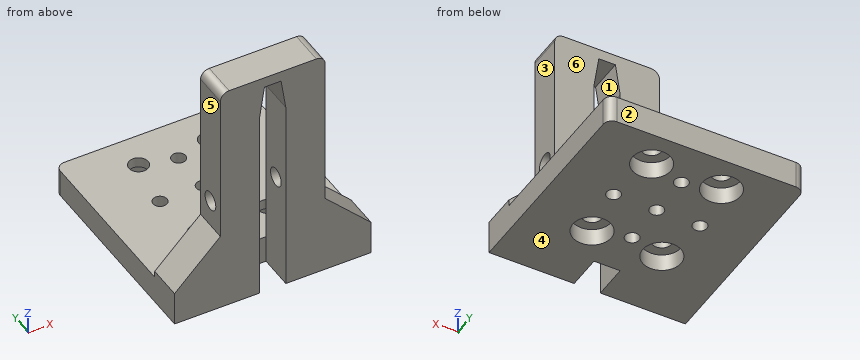
from build123d import *

# Parameters (mm, degrees)
SKETCH1_W                      = 22.5
SKETCH1_H                      = 20
BOSS_EXTRUDE1_DEPTH            = 3.175
TAP_DRILL_FOR_M2X0_4_TAP2_D    = 1.6
BOSS_EXTRUDE2_DEPTH            = 4
CHAMFER1_SIZE                  = 6
M2_CLEARANCE_HOLE1_D           = 2.15
FILLET1_R                      = 1
CBORE_FOR_M2_SHCS1_D           = 2.2
CBORE_FOR_M2_SHCS1_CBORE_D     = 4.4
CBORE_FOR_M2_SHCS1_CBORE_DEPTH = 2


with BuildPart() as part:
    # Sketch1 → Boss-Extrude1 (new body)
    with BuildSketch(Plane.XY):
        Rectangle(SKETCH1_W, SKETCH1_H)
    extrude(amount=BOSS_EXTRUDE1_DEPTH)

    # Tap Drill for M2x0.4 Tap2 (through all)
    with Locations(Plane.XY.offset(3.175)):
        with Locations((0, 0), (-4.949747468, 0), (0, -4.949747468), (4.949747468, 0), (0, 4.949747468)):
            Hole(TAP_DRILL_FOR_M2X0_4_TAP2_D / 2)

    # Sketch10 → Boss-Extrude2 (add)
    with BuildSketch(Plane.XZ.offset(10)):
        Polygon((6, 27.65), (-6, 27.65), (-6, 3.175), (-11.25, 3.175), (-11.25, 0), (-1.5, 0), (-1.5, 22.8), (-0.95, 26.45), (0.95, 26.45), (1.5, 22.8), (1.5, 0), (11.25, 0), (11.25, 3.175), (6, 3.175), align=None)
    extrude(amount=BOSS_EXTRUDE2_DEPTH)

    # Chamfer1
    # the kernel refuses this chamfer: 6 mm, written as the material it adds along each edge
    with BuildSketch(Plane(origin=(-6, -10, 3.175), x_dir=(-0.9996219169112969, 0, -0.02749587661058649), z_dir=(0, -1, 0))) as chamfer1_piece_1_section:
        Polygon((CHAMFER1_SIZE * 0.999621916911, -CHAMFER1_SIZE * 0.0274958766106), (-CHAMFER1_SIZE * 0.0274958766106, -CHAMFER1_SIZE * 0.999621916911), (0, 0), align=None)
    chamfer1_piece_1 = extrude(amount=4, mode=Mode.PRIVATE)
    chamfer1_piece_1 = split(chamfer1_piece_1, bisect_by=Plane(origin=(-11.25, -12, 5.202939), z_dir=(1, 0, 0)), keep=Keep.TOP, mode=Mode.PRIVATE)
    add(chamfer1_piece_1)
    with BuildSketch(Plane(origin=(6, -10, 3.175), x_dir=(0.9996219169112969, 0, -0.02749587661058649), z_dir=(0, -1, 0))) as chamfer1_piece_2_section:
        Polygon((CHAMFER1_SIZE * 0.999621916911, CHAMFER1_SIZE * 0.0274958766106), (-CHAMFER1_SIZE * 0.0274958766106, CHAMFER1_SIZE * 0.999621916911), (0, 0), align=None)
    chamfer1_piece_2 = extrude(amount=4, mode=Mode.PRIVATE)
    chamfer1_piece_2 = split(chamfer1_piece_2, bisect_by=Plane(origin=(11.25, -12, 5.202939), z_dir=(-1, 0, 0)), keep=Keep.TOP, mode=Mode.PRIVATE)
    add(chamfer1_piece_2)

    # M2 Clearance Hole1 (through all)
    with Locations(Plane.ZY.offset(11.25)):
        with Locations((12.35, -12)):
            Hole(M2_CLEARANCE_HOLE1_D / 2)

    # Fillet1
    fillet1_edges = [part.edges().sort_by_distance(p)[0] for p in [
        (6, -12, 27.65),
        (-6, -12, 27.65),
        (-11.25, 10, 1.5875),
        (11.25, 10, 1.5875),
    ]]
    fillet(fillet1_edges, radius=FILLET1_R)

    # CBORE for M2 SHCS1 (through all)
    with Locations(Plane(origin=(0, 0, 0), x_dir=(-1, 0, 0), z_dir=(0, 0, -1))):
        with Locations((4, -6), (-4, 6), (-4, -6), (4, 6)):
            CounterBoreHole(CBORE_FOR_M2_SHCS1_D / 2, CBORE_FOR_M2_SHCS1_CBORE_D / 2, CBORE_FOR_M2_SHCS1_CBORE_DEPTH)


solid = part.part
For this review, take the finished solid that the model builds, in its own axes (mm). Face numbers are marked on the shaded views. A direction names the side the tool comes from. Round coordinates to 2 decimals unless told otherwise and drop trailing zeros. Loops run counter-clockwise (first coordinate to the right, second up) from the corner with the lowest first, then second, coordinate; pieces in that order, holes last. Notation, with made-up numbers: (3.25, -4) - (23.25, -4) arc R11 cw to (23.25, 9) - close; hole circle Ø1 at (55.25, -16.75). An arc over 180 degrees is marked (long way). One line per question, with ' | ' between items.
Q1. The part is to be moulded in two halves that separate along X. For the marked faces 1, 2 and 3, say which applies: released by +X, released by -X, zero draft, split by the parting line, or undercut.
Taken from the geometry:
face 1: undercut | face 2: zero draft | face 3: released by +X
Q2. For pin 1 (1.2 mm diameter, centred on y = -11, z = 17, fed in from +X); pin 2 (3.5 mm diameter, centred on x = 4, y = 6, fed in from -Z); pin 3 (1.8 mm diameter, centred on x = -4, y = -6, fed in from -Z); pin 4 (2.5 mm diameter, centred on x = -4, y = 6, fed in from +Z) (3 decimals), all flat-tipped, find the tip position at first contact; note any pin that passes through.
Taken from the geometry:
pin 1: stops at x = 6 | pin 2: stops at z = 2 | pin 3: passes through | pin 4: stops at z = 3.175
Q3. For line 1 along Y through (x, z) = (4, 2.7); line 2 along Y through (x, z) = (4, 0.75); line 3 along Z through (x, y) = (1, -8) (3 decimals), list the stretches that pass through material, from the lowest coordinate up. Write a range as [from, to].
Taken from the geometry:
line 1: y = [-14, -7.1], [-4.9, 4.9], [7.1, 10] | line 2: y = [-14, -8.2], [-3.8, 3.8], [8.2, 10] | line 3: z = [0, 3.175]
Q4. Tool access review of the marked faces 4, 5 and 6: name each direction out of +Z, -Z, +X, -X, +Y, -Y from which nothing blocks a thin tool from reaching the whole face with its end or side.
Taken from the geometry:
face 4: -Z, +X, -X, +Y, -Y | face 5: +Z, -X, +Y, -Y | face 6: +Z, +X, -X, +Y
Q5. Take a section at D-D (z = 5.5). Give the boundary of the cut face in (x, y) (3 decimals).
Taken from the geometry:
outline: (-9.675, -14) - (-1.5, -14) - (-1.5, -10) - (-9.675, -10) - close; (1.5, -14) - (9.675, -14) - (9.675, -10) - (1.5, -10) - close
Q6. Take a section at B-B (y = -12). Give the boundary of the cut face in (x, z) (3 decimals).
Taken from the geometry:
outline: (-11.25, 0) - (-1.5, 0) - (-1.5, 11.275) - (-6, 11.275) - (-6, 9.175) - (-11.25, 3.925) - close; (-6, 13.425) - (-1.5, 13.425) - (-1.5, 22.8) - (-0.95, 26.45) - (0.95, 26.45) - (1.5, 22.8) - (1.5, 13.425) - (6, 13.425) - (6, 26.65) arc R1 ccw to (5, 27.65) - (-5, 27.65) arc R1 ccw to (-6, 26.65) - close; (1.5, 0) - (11.25, 0) - (11.25, 3.925) - (6, 9.175) - (6, 11.275) - (1.5, 11.275) - close
Q7. Take a section at C-C (x = 0). Give the boundary of the cut face in (y, z) (3 decimals).
Taken from the geometry:
outline: (-14, 26.45) - (-10, 26.45) - (-10, 27.65) - (-14, 27.65) - close; (-10, 0) - (-5.75, 0) - (-5.75, 3.175) - (-10, 3.175) - close; (-4.15, 0) - (-0.8, 0) - (-0.8, 3.175) - (-4.15, 3.175) - close; (0.8, 0) - (4.15, 0) - (4.15, 3.175) - (0.8, 3.175) - close; (5.75, 0) - (10, 0) - (10, 3.175) - (5.75, 3.175) - close
Q8. Take a section at A-A (z = 12.35). Give the boundary of the cut face in (x, y) (3 decimals), and give its area (4 significant figures).
Taken from the geometry:
outline: (-6, -14) - (-1.5, -14) - (-1.5, -13.075) - (-6, -13.075) - close; (-6, -10.925) - (-1.5, -10.925) - (-1.5, -10) - (-6, -10) - close; (1.5, -14) - (6, -14) - (6, -13.075) - (1.5, -13.075) - close; (1.5, -10.925) - (6, -10.925) - (6, -10) - (1.5, -10) - close | area: 16.65 mm²
